Could you check a few things on this model? Use its own coordinates, in mm. A direction names the side the tool comes from. Coordinates: 2 decimals unless noted, no trailing zeros. Loops run counter-clockwise (first coordinate to the right, second up) from the corner with the lowest first, then second, coordinate; pieces in that order, holes last.
from build123d import *

# Parameters (mm, degrees)
F0_W     = 170
F0_H     = 68
F1_DEPTH = 60
F2_R     = 4
F3_DEPTH = 10


with BuildPart() as f1:
    # F0 (on Top) → F1 (new body)
    with BuildSketch(Plane.XY):
        Rectangle(F0_W, F0_H)
    extrude(amount=F1_DEPTH)

    # F2 (on face) → F3 (join)
    with BuildSketch(Plane(origin=(-85, 0, 0), x_dir=(0, -1, 0), z_dir=(-1, 0, 0))):
        with Locations((4.5, 56)):
            Circle(F2_R)
        with Locations((-4.5, 56)):
            Circle(F2_R)
    extrude(amount=F3_DEPTH)


solid = f1.part
(1) We'd pull the mould along Y, two halves only. Please class faces 3 (the face through (-1, 34, 30)), 4 (the face through (-89.93, -3.633, 52.095)), 5 (the face through (-95, -4, 56)): +Y half, -Y half, draft (parallel to the pull), parting line (faces both ways), or undercut.
Answers:
face 3: +Y half
face 4: undercut
face 5: draft
(2) Which directions (+Z, -Z, +X, -X, +Y, -Y) give clear straight access to the entire face, cutting with the end or side of a thin tool? Please do faces 1 (the face through (-89.93, 5.367, 52.095)), 2 (the face through (-95, 5, 56)).
Answers:
face 1: -X
face 2: +Z, -Z, -X, +Y, -Y
(3) Imagine slicing it at B-B, the plane y = -22. Write out the boundary of the cut face in (x, z), and give its area (3 significant figures).
Answers:
outline: (-85, 0) - (85, 0) - (85, 60) - (-85, 60) - close
area: 10,200 mm2
(4) I need wall thicknesses on probe 1 along X at (y, z) = (-17.5, 28). Which ranges of the line are inside material? Lowest first, please.
Answers:
probe 1: x = -85 to 85
(5) Imagine slicing it at A-A, the plane z = 56. Write out the boundary of the cut face in (x, y).
Answers:
outline: (-95, -8.5) - (-85, -8.5) - (-85, -34) - (85, -34) - (85, 34) - (-85, 34) - (-85, 8.5) - (-95, 8.5) - (-95, 0.5) - (-85, 0.5) - (-85, -0.5) - (-95, -0.5) - close
(6) For pin 1 (2 mm diameter, centred on y = -25, z = 22, fed in from -X), with a flat end and sliding along its axis, tell me the tip position at first contact or that it passes through.
Answers:
pin 1: stops at x = -85
(7) Imagine slicing it at C-C, the plane z = 38. Write out the boundary of the cut face in (x, y).
Answers:
outline: (-85, -34) - (85, -34) - (85, 34) - (-85, 34) - close
